Verification items for the finished model (mm, model axes). A direction names the side the tool comes from. Give positions to 0.01 mm unless a question says otherwise; leave off trailing zeros. Loops run counter-clockwise (first coordinate to the right, second up) from the corner with the lowest first, then second, coordinate; pieces in that order, holes last. Notation, with made-up numbers: M -5,28 L 16,28 A31 ccw 16,61 Z; hole C 14,39 d9. An arc over 180 degrees is marked long. Use CSV: the item, a comma, the result in double quotes.
from build123d import *

# Parameters (mm, degrees)
PAD_DEPTH    = 3
CHAMFER_SIZE = 2
FILLET_R     = 2


with BuildPart() as part:
    # Sketch → Pad (new body)
    with BuildSketch(Plane.XY):
        with BuildLine():
            ThreePointArc((-25.475478, -24), (0, -35), (25.475478, -24))
            Line((25.475478, -24), (38.065733, -24))
            ThreePointArc((4, -44.82187), (23.468469, -38.395716), (38.065733, -24))
            Line((0, -48), (4, -44.82187))
            Line((0, -48), (0, -55))
            Line((0, -55), (-20, -55))
            Line((-20, -55), (-20, -48))
            Line((-24, -38.065733), (-20, -48))
            ThreePointArc((-38.065733, -24), (-31.819805, -31.819805), (-24, -38.065733))
            Line((-25.475478, -24), (-38.065733, -24))
        make_face()
        with BuildLine():
            ThreePointArc((-30.034271, -26.084271), (-32.234271, -28.284271), (-30.034271, -30.484271))
            Line((-30.034271, -30.484271), (-26.534271, -30.484271))
            ThreePointArc((-26.534271, -30.484271), (-24.334271, -28.284271), (-26.534271, -26.084271))
            Line((-30.034271, -26.084271), (-26.534271, -26.084271))
        make_face(mode=Mode.SUBTRACT)
        with BuildLine():
            ThreePointArc((26.534271, -26.084271), (24.334271, -28.284271), (26.534271, -30.484271))
            Line((26.534271, -30.484271), (30.034271, -30.484271))
            ThreePointArc((30.034271, -30.484271), (32.234271, -28.284271), (30.034271, -26.084271))
            Line((26.534271, -26.084271), (30.034271, -26.084271))
        make_face(mode=Mode.SUBTRACT)
        with BuildLine():
            ThreePointArc((-4.25, -44.5), (-5.5, -43.25), (-6.75, -44.5))
            Line((-6.75, -44.5), (-6.75, -47.5))
            ThreePointArc((-6.75, -47.5), (-5.5, -48.75), (-4.25, -47.5))
            Line((-4.25, -44.5), (-4.25, -47.5))
        make_face(mode=Mode.SUBTRACT)
        with BuildLine():
            ThreePointArc((-13.75, -44.5), (-15, -43.25), (-16.25, -44.5))
            Line((-16.25, -44.5), (-16.25, -47.5))
            ThreePointArc((-16.25, -47.5), (-15, -48.75), (-13.75, -47.5))
            Line((-13.75, -44.5), (-13.75, -47.5))
        make_face(mode=Mode.SUBTRACT)
    extrude(amount=PAD_DEPTH)

    # Chamfer
    chamfer_edges = [part.edges().sort_by_distance(p)[0] for p in [
        (0, -55, 1.5),
        (38.065733, -24, 1.5),
        (-38.065733, -24, 1.5),
        (-20, -55, 1.5),
    ]]
    chamfer(chamfer_edges, length=CHAMFER_SIZE)

    # Fillet
    fillet_edges = [part.edges().sort_by_distance(p)[0] for p in [
        (-20, -48, 1.5),
        (-24, -38.065733, 1.5),
        (0, -48, 1.5),
        (4, -44.82187, 1.5),
    ]]
    fillet(fillet_edges, radius=FILLET_R)


solid = part.part
(1) Scan lines: L1, parallel to X at y = -45, z = 1.3; L2, parallel to Y at x = 29.5, z = 1.5; L3, parallel to X at y = -27.5, z = 1.2. Record each from-to range of solid material in increasing order. Write a range as from..to.
Calculated:
L1,"x = -21.21..-16.25, -13.75..-6.75, -4.25..3.82"
L2,"y = -33.98..-30.48, -26.08..-24"
L3,"x = -35.62..-32.09, -24.48..-21.65, 21.65..24.48, 32.09..35.62"
(2) Tool access check on faces 1 (the flat face through (1, -36, 3)), 2 (the flat face through (-28, -30.484, 1)). Record the directions out of +Z, -Z, +X, -X, +Y, -Y that give a thin tool (end or side, any length) a straight path to the whole face; none if there is none.
Calculated:
face 1,"+Z, +X, -X, +Y, -Y"
face 2,"+Z, -Z"
(3) Section check C-C on x = -5.5. Record the cut outline in (y, z), plus the area to 3 significant figures.
Calculated:
outline,"M -55,0 L -48.75,0 L -48.75,3 L -55,3 Z; M -43.25,0 L -34.57,0 L -34.57,3 L -43.25,3 Z"
area,"44.8 mm²"
(4) Section check B-B on y = -31.5. Record the cut outline in (x, z).
Calculated:
outline,"M -32.14,0 L -15.26,0 L -15.26,3 L -32.14,3 Z; M 15.26,0 L 32.14,0 L 32.14,3 L 15.26,3 Z"
(5) Section check A-A on z = 2.25. Count the separate pieces of the cut face and the enclosed holes in it, plus the area to 3 significant figures.
Calculated:
separate pieces,"1"
enclosed holes,"4"
area,"899 mm²"
(6) Section check D-D on x = -23. Record the cut outline in (y, z), plus the area to 3 significant figures.
Calculated:
outline,"M -40.55,0 L -26.38,0 L -26.38,3 L -40.55,3 Z"
area,"42.5 mm²"
(7) Depth check by flat-ended pin: pin 1 Ø1.5 at (x, z) = (-28.5, 1.5) entering from -Y; pin 2 Ø1.5 at (y, z) = (-50.5, 2) entering from +X; pin 3 Ø0.9 at (y, z) = (-46, 1) entering from -X; pin 4 Ø6 at (x, y) = (-3, -32) entering from +Z. Enter the tip coordinate at first touch or a pass-through.
Calculated:
pin 1,"stops at y = -35.43"
pin 2,"stops at x = 0"
pin 3,"stops at x = -20.99"
pin 4,"stops at z = 3"
(8) Mould release check, pull along X, two halves, no side actions. Record for faces 3 (the flat face through (-21.978, -43.087, 1.479)), 4 (the flat face through (36.52, -24.846, 1.479)), 5 (the cylindrical face through (-5.53, -48.75, 1.48)): released by +X, released by -X, zero draft, split by the parting line, or undercut.
Calculated:
face 3,"released by -X"
face 4,"released by +X"
face 5,"undercut"
